Design review of the part built by this model. Coordinates are the model's own, in mm. Give positions to 0.01 mm unless a question says otherwise; leave off trailing zeros. Loops run counter-clockwise (first coordinate to the right, second up) from the corner with the lowest first, then second, coordinate; pieces in that order, holes last. Notation, with made-up numbers: (-15.75, 58.25) -> (14.25, 58.25) arc R27 cw to (14.25, 77.25) -> close; hole circle Ø10 at (44.5, 55.25). An arc over 180 degrees is marked (long way). Answer as CSV lines item,"result".
from build123d import *

# Parameters (mm, degrees)
CHAMFER1_SIZE                  = 1
CHAMFER1_SIZE2                 = 2.747477419
CIRPATTERN2_COUNT              = 3
BOSS_EXTRUDE1_DEPTH            = 3
SKETCH4_R                      = 7.5
CUT_EXTRUDE1_DEPTH             = 49.603797643
SKETCH6_W                      = 1.25
SKETCH6_H                      = 3
M3X0_5_TAPPED_HOLE2_AT_2_COUNT = 2
M3X0_5_TAPPED_HOLE2_AT_2_PITCH = 20.784609691
M3X0_5_TAPPED_HOLE2_AT_3_COUNT = 2
M3X0_5_TAPPED_HOLE2_AT_3_PITCH = 20.784609691
FILLET1_R                      = 5
FILLET2_R                      = 2
SKETCH9_W                      = 1.6
SKETCH9_H                      = 6.6
M3_CLEARANCE_HOLE3_AT_2_COUNT  = 2
M3_CLEARANCE_HOLE3_AT_2_PITCH  = 14
M3_CLEARANCE_HOLE3_AT_3_COUNT  = 2
M3_CLEARANCE_HOLE3_AT_3_PITCH  = 28
M3_CLEARANCE_HOLE3_AT_4_COUNT  = 2
M3_CLEARANCE_HOLE3_AT_4_PITCH  = 50.5
M3_CLEARANCE_HOLE3_AT_5_COUNT  = 2
M3_CLEARANCE_HOLE3_AT_5_PITCH  = 57.742964939
M3_CLEARANCE_HOLE3_AT_6_COUNT  = 2
M3_CLEARANCE_HOLE3_AT_6_PITCH  = 39.597979746
M3_CLEARANCE_HOLE3_AT_7_COUNT  = 2
M3_CLEARANCE_HOLE3_AT_7_PITCH  = 31.304951685
M3_CLEARANCE_HOLE3_AT_8_COUNT  = 2
M3_CLEARANCE_HOLE3_AT_8_PITCH  = 28
SKETCH13_W                     = 1.6
SKETCH13_H                     = 6.6
M3_CLEARANCE_HOLE2_AT_2_COUNT  = 2
M3_CLEARANCE_HOLE2_AT_2_PITCH  = 51.961524227
M3_CLEARANCE_HOLE2_AT_3_COUNT  = 2
M3_CLEARANCE_HOLE2_AT_3_PITCH  = 51.961524227
CHAMFER2_SIZE                  = 0.4
CHAMFER3_SIZE                  = 0.4
CHAMFER4_SIZE                  = 0.4


with BuildPart() as part:
    # Sketch3 → Revolve1 (revolve)
    with BuildSketch(Plane(origin=(0, 0, 0), x_dir=(0, 0, -1), z_dir=(1, 0, 0)), mode=Mode.PRIVATE) as revolve1_sk:
        with BuildLine():
            Line((0, 31.6), (0.233939444, 31.6))
            ThreePointArc((0.233939444, 31.6), (1.585065492, 33.262066557), (3.6, 33.988734135))
            Line((3.6, 33.988734135), (3.6, 35.988734135))
            Line((3.6, 35.988734135), (0, 35.988734135))
            Line((0, 35.988734135), (0, 31.6))
        make_face()
    revolve(revolve1_sk.sketch.rotate(Axis((0, 30, 0), (0, 0, -1)), 90), axis=Axis((0, 30, 0), (0, 0, -1)))

    # Chamfer1
    chamfer1_edges = [part.edges().sort_by_distance(p)[0] for p in [
        (-5.988734135, 30, -3.6),
    ]]
    chamfer1_side = [part.faces().sort_by_distance(p)[0] for p in [
        (-4.158121116, 30, -3.6),
    ]]
    chamfer(chamfer1_edges, length=CHAMFER1_SIZE, length2=CHAMFER1_SIZE2, reference=chamfer1_side[0])


with BuildPart() as cirpattern2_1:
    # CirPattern2: pattern copy
    add(part.part.rotate(Axis((0, 0, 0), (0, 0, 1)), 1 * 360 / CIRPATTERN2_COUNT))

    # Chamfer4
    # the kernel refuses this chamfer: 0.4 mm, written as the material it takes off along each edge
    with BuildSketch(Plane(origin=(-25.980762114, -15, 0), x_dir=(-0.5000000000000001, 0.8660254037844387, 0), z_dir=(-0.8660254037844387, -0.5000000000000001, 0))) as chamfer4_piece_1:
        Polygon((5.988734135, CHAMFER4_SIZE), (5.988734135 - CHAMFER4_SIZE, 0), (5.988734135, 0), align=None)
    revolve(axis=Axis((-25.980762114, -15, 0), (0, 0, -1)), mode=Mode.SUBTRACT)
    with BuildSketch(Plane(origin=(-25.980762114, -15, 0), x_dir=(-0.4999999999999992, 0.866025403784439, 0), z_dir=(-0.866025403784439, -0.4999999999999992, 0))) as chamfer4_piece_2:
        Polygon((1.6, CHAMFER4_SIZE), (1.6 + CHAMFER4_SIZE, 0), (1.6, 0), align=None)
    revolve(axis=Axis((-25.980762114, -15, 0), (0, 0, -1)), mode=Mode.SUBTRACT)


with BuildPart() as cirpattern2_2:
    # CirPattern2: pattern copy
    add(part.part.rotate(Axis((0, 0, 0), (0, 0, 1)), 2 * 360 / CIRPATTERN2_COUNT))

    # Chamfer2
    # the kernel refuses this chamfer: 0.4 mm, written as the material it takes off along each edge
    with BuildSketch(Plane(origin=(25.980762114, -15, 0), x_dir=(-0.5000000000000006, -0.8660254037844384, 0), z_dir=(0.8660254037844384, -0.5000000000000006, 0))) as chamfer2_piece_1:
        Polygon((5.988734135, CHAMFER2_SIZE), (5.988734135 - CHAMFER2_SIZE, 0), (5.988734135, 0), align=None)
    revolve(axis=Axis((25.980762114, -15, 0), (0, 0, -1)), mode=Mode.SUBTRACT)
    with BuildSketch(Plane(origin=(25.980762114, -15, 0), x_dir=(-0.5000000000000004, -0.8660254037844384, 0), z_dir=(0.8660254037844384, -0.5000000000000004, 0))) as chamfer2_piece_2:
        Polygon((1.6, CHAMFER2_SIZE), (1.6 + CHAMFER2_SIZE, 0), (1.6, 0), align=None)
    revolve(axis=Axis((25.980762114, -15, 0), (0, 0, -1)), mode=Mode.SUBTRACT)


with BuildPart() as body_4:
    # Sketch1 → Boss-Extrude1 (new body)
    with BuildSketch(Plane.XY):
        with BuildLine():
            Line((25.980762114, -21), (-25.980762114, -21))
            ThreePointArc((-25.980762114, -21), (-31.776317071, -16.552914271), (-28.980762114, -9.803847577))
            Line((-28.980762114, -9.803847577), (-17.5, -3.175426481))
            Line((-17.5, -3.175426481), (-17.5, 36))
            Line((-17.5, 36), (17.5, 36))
            Line((17.5, 36), (17.5, -3.175426481))
            Line((17.5, -3.175426481), (28.980762114, -9.803847577))
            ThreePointArc((28.980762114, -9.803847577), (31.776317071, -16.552914271), (25.980762114, -21))
        make_face()
    extrude(amount=BOSS_EXTRUDE1_DEPTH)

    # Sketch4 → Cut-Extrude1 (cut, through all)
    with BuildSketch(Plane.XY.offset(3)):
        Circle(SKETCH4_R)
    extrude(amount=-CUT_EXTRUDE1_DEPTH, mode=Mode.SUBTRACT)

    # Sketch6 → M3x0.5 Tapped Hole2 (revolve, cut)
    with BuildSketch(Plane(origin=(-10.392304845, -6, 0), x_dir=(0, 1, 0), z_dir=(1, 0, 0))):
        with Locations((0.625, 1.5)):
            Rectangle(SKETCH6_W, SKETCH6_H)
    m3x0_5_tapped_hole2 = revolve(axis=Axis((-10.392304845, -6, -6.35), (0, 0, 1)), mode=Mode.SUBTRACT)

    # M3x0.5 Tapped Hole2 at 2: M3x0.5 Tapped Hole2 ×2
    with Locations(*[Vector(0.49999999999999795, 0.8660254037844399, 0) * (i * M3X0_5_TAPPED_HOLE2_AT_2_PITCH) for i in range(1, M3X0_5_TAPPED_HOLE2_AT_2_COUNT)]):
        add(m3x0_5_tapped_hole2, mode=Mode.SUBTRACT)

    # M3x0.5 Tapped Hole2 at 3: M3x0.5 Tapped Hole2 ×2
    with Locations(*[(i * M3X0_5_TAPPED_HOLE2_AT_3_PITCH, 0, 0) for i in range(1, M3X0_5_TAPPED_HOLE2_AT_3_COUNT)]):
        add(m3x0_5_tapped_hole2, mode=Mode.SUBTRACT)

    # Fillet1
    fillet1_edges = [body_4.edges().sort_by_distance(p)[0] for p in [
        (-17.5, -3.175426481, 1.5),
        (17.5, -3.175426481, 1.5),
    ]]
    fillet(fillet1_edges, radius=FILLET1_R)

    # Fillet2
    fillet2_edges = [body_4.edges().sort_by_distance(p)[0] for p in [
        (-17.5, 36, 1.5),
        (17.5, 36, 1.5),
    ]]
    fillet(fillet2_edges, radius=FILLET2_R)

    # Sketch9 → M3 Clearance Hole3 (revolve, cut)
    with BuildSketch(Plane(origin=(14, 32.5, 3), x_dir=(0, -1, 0), z_dir=(1, 0, 0))):
        with Locations((0.8, 3.3)):
            Rectangle(SKETCH9_W, SKETCH9_H)
    m3_clearance_hole3 = revolve(axis=Axis((14, 32.5, 9.35), (0, 0, -1)), mode=Mode.SUBTRACT)

    # M3 Clearance Hole3 at 2: M3 Clearance Hole3 ×2
    with Locations(*[(0, -i * M3_CLEARANCE_HOLE3_AT_2_PITCH, 0) for i in range(1, M3_CLEARANCE_HOLE3_AT_2_COUNT)]):
        add(m3_clearance_hole3, mode=Mode.SUBTRACT)

    # M3 Clearance Hole3 at 3: M3 Clearance Hole3 ×2
    with Locations(*[(0, -i * M3_CLEARANCE_HOLE3_AT_3_PITCH, 0) for i in range(1, M3_CLEARANCE_HOLE3_AT_3_COUNT)]):
        add(m3_clearance_hole3, mode=Mode.SUBTRACT)

    # M3 Clearance Hole3 at 4: M3 Clearance Hole3 ×2
    with Locations(*[(0, -i * M3_CLEARANCE_HOLE3_AT_4_PITCH, 0) for i in range(1, M3_CLEARANCE_HOLE3_AT_4_COUNT)]):
        add(m3_clearance_hole3, mode=Mode.SUBTRACT)

    # M3 Clearance Hole3 at 5: M3 Clearance Hole3 ×2
    with Locations(*[Vector(-0.48490755591360857, -0.8745654133441881, 0) * (i * M3_CLEARANCE_HOLE3_AT_5_PITCH) for i in range(1, M3_CLEARANCE_HOLE3_AT_5_COUNT)]):
        add(m3_clearance_hole3, mode=Mode.SUBTRACT)

    # M3 Clearance Hole3 at 6: M3 Clearance Hole3 ×2
    with Locations(*[Vector(-0.7071067811865479, -0.7071067811865472, 0) * (i * M3_CLEARANCE_HOLE3_AT_6_PITCH) for i in range(1, M3_CLEARANCE_HOLE3_AT_6_COUNT)]):
        add(m3_clearance_hole3, mode=Mode.SUBTRACT)

    # M3 Clearance Hole3 at 7: M3 Clearance Hole3 ×2
    with Locations(*[Vector(-0.8944271909999161, -0.4472135954999577, 0) * (i * M3_CLEARANCE_HOLE3_AT_7_PITCH) for i in range(1, M3_CLEARANCE_HOLE3_AT_7_COUNT)]):
        add(m3_clearance_hole3, mode=Mode.SUBTRACT)

    # M3 Clearance Hole3 at 8: M3 Clearance Hole3 ×2
    with Locations(*[(-i * M3_CLEARANCE_HOLE3_AT_8_PITCH, 0, 0) for i in range(1, M3_CLEARANCE_HOLE3_AT_8_COUNT)]):
        add(m3_clearance_hole3, mode=Mode.SUBTRACT)

    # Sketch13 → M3 Clearance Hole2 (revolve, cut)
    with BuildSketch(Plane(origin=(0, 30, 3), x_dir=(0, -1, 0), z_dir=(1, 0, 0))):
        with Locations((0.8, 3.3)):
            Rectangle(SKETCH13_W, SKETCH13_H)
    m3_clearance_hole2 = revolve(axis=Axis((0, 30, 9.35), (0, 0, -1)), mode=Mode.SUBTRACT)

    # M3 Clearance Hole2 at 2: M3 Clearance Hole2 ×2
    with Locations(*[Vector(0.49999999999999795, -0.8660254037844398, 0) * (i * M3_CLEARANCE_HOLE2_AT_2_PITCH) for i in range(1, M3_CLEARANCE_HOLE2_AT_2_COUNT)]):
        add(m3_clearance_hole2, mode=Mode.SUBTRACT)

    # M3 Clearance Hole2 at 3: M3 Clearance Hole2 ×2
    with Locations(*[Vector(-0.49999999999999784, -0.8660254037844399, 0) * (i * M3_CLEARANCE_HOLE2_AT_3_PITCH) for i in range(1, M3_CLEARANCE_HOLE2_AT_3_COUNT)]):
        add(m3_clearance_hole2, mode=Mode.SUBTRACT)


with BuildPart() as part_1:
    add(part.part)

    # Chamfer3
    # the kernel refuses this chamfer: 0.4 mm, written as the material it takes off along each edge
    with BuildSketch(Plane(origin=(0, 30, 0), x_dir=(1, 0, 0), z_dir=(0, 1, 0))) as chamfer3_piece_1:
        Polygon((5.988734135, CHAMFER3_SIZE), (5.988734135 - CHAMFER3_SIZE, 0), (5.988734135, 0), align=None)
    revolve(axis=Axis((0, 30, 0), (0, 0, -1)), mode=Mode.SUBTRACT)
    with BuildSketch(Plane(origin=(0, 30, 0), x_dir=(1, 0, 0), z_dir=(0, 1, 0))) as chamfer3_piece_2:
        Polygon((1.6, CHAMFER3_SIZE), (1.6 + CHAMFER3_SIZE, 0), (1.6, 0), align=None)
    revolve(axis=Axis((0, 30, 0), (0, 0, -1)), mode=Mode.SUBTRACT)


solid = body_4.part
Q1. We need section A-A, the plane x = 6. State the section outline as (y, z) points, and give its area (3 significant figures).
Filled sheet:
outline,"(-21, 0) -> (-4.5, 0) -> (-4.5, 3) -> (-21, 3) -> close; (4.5, 0) -> (36, 0) -> (36, 3) -> (4.5, 3) -> close"
area,"144 mm^2"
Q2. Clearance check with flat-ended pins moving along their axes: pin 1 Ø1 at (y, z) = (4, 1) entering from +X; pin 2 Ø1.5 at (y, z) = (13.5, 1.5) entering from -X. State where each tip first meets the part, or that it passes through.
Filled sheet:
pin 1,"stops at x = 17.5"
pin 2,"stops at x = -17.5"
Q3. To check wall thickness, follow probe 1 along X at (y, z) = (-15, 2.1); probe 2 along Y at (x, z) = (14, 1.25); probe 3 along Y at (x, z) = (13, 1.3). State the ranges of each line that lie inside material, in increasing order. Write a range as from..to.
Filled sheet:
probe 1,"x = -31.98..-27.58, -24.38..24.38, 27.58..31.98"
probe 2,"y = -21..-19.6, -16.4..2.9, 6.1..16.9, 20.1..30.9, 34.1..36"
probe 3,"y = -21..-19.25, -16.75..3.25, 5.75..17.25, 19.75..31.25, 33.75..36"
Q4. We need section B-B, the plane y = -15. State the section outline as (x, z) points.
Filled sheet:
outline,"(-31.98, 0) -> (-27.58, 0) -> (-27.58, 3) -> (-31.98, 3) -> close; (-24.38, 0) -> (24.38, 0) -> (24.38, 3) -> (-24.38, 3) -> close; (27.58, 0) -> (31.98, 0) -> (31.98, 3) -> (27.58, 3) -> close"
Q5. The part is to be moulded in two halves that separate along X. For faces 1 (the flat face through (0, 8, 3)), 2 (the cylindrical face through (12.92, 19.68, 1.48)), 3 (the flat face through (24.428, -7.175, 1.479)), say which applies: pulls with the +X half, pulls with the -X half, needs draft (parallel to the pull), parting line crosses it, or undercut.
Filled sheet:
face 1,"needs draft"
face 2,"undercut"
face 3,"pulls with the +X half"
Q6. We need section D-D, the plane y = -6. State the section outline as (x, z) points, and give its area (3 significant figures).
Filled sheet:
outline,"(-22.39, 0) -> (-11.64, 0) -> (-11.64, 3) -> (-22.39, 3) -> close; (-9.14, 0) -> (-4.5, 0) -> (-4.5, 3) -> (-9.14, 3) -> close; (4.5, 0) -> (9.14, 0) -> (9.14, 3) -> (4.5, 3) -> close; (11.64, 0) -> (22.39, 0) -> (22.39, 3) -> (11.64, 3) -> close"
area,"92.4 mm^2"
Q7. We need section C-C, the plane x = -14. State the section outline as (y, z) points.
Filled sheet:
outline,"(-21, 0) -> (-19.6, 0) -> (-19.6, 3) -> (-21, 3) -> close; (-16.4, 0) -> (2.9, 0) -> (2.9, 3) -> (-16.4, 3) -> close; (6.1, 0) -> (16.9, 0) -> (16.9, 3) -> (6.1, 3) -> close; (20.1, 0) -> (30.9, 0) -> (30.9, 3) -> (20.1, 3) -> close; (34.1, 0) -> (36, 0) -> (36, 3) -> (34.1, 3) -> close"
